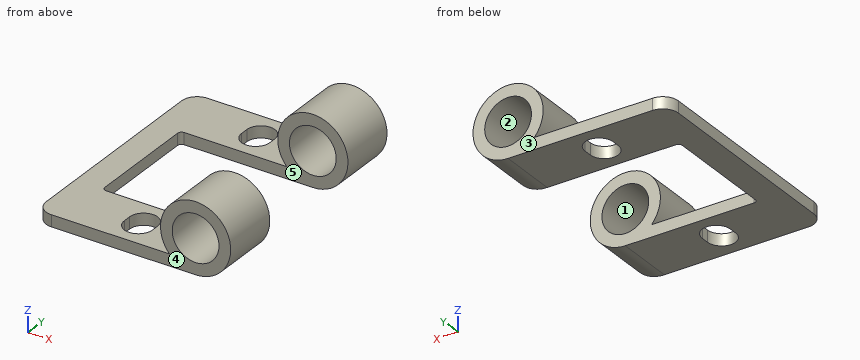
from build123d import *

# Parameters (mm, degrees)
SKETCH_2_W             = 16
SKETCH_2_H             = 30
SM_BASE_FLANGE_1_DEPTH = 1.5
SKETCH_7_R             = 4.5
SKETCH_7_R_2           = 3
EXTRUDE_1_DEPTH        = 30
SKETCH_8_W             = 1.5
SKETCH_8_H             = 7.5
EXTRUDE_1_2_DEPTH      = 4.5
SKETCH_9_W             = 25
SKETCH_9_H             = 15
CUT_EXTRUDE_1_DEPTH    = 41.074929819
FILLET_1_R             = 2
CUT_EXTRUDE_2_DEPTH    = 10
FILLET_2_R             = 0.5


# Sheet-metal steps are written as plain solids
with BuildPart() as part:
    # Sketch 2 → Базовая кромка1 (new body)
    with BuildSketch(Plane.XY):
        with Locations((8, -15)):
            Rectangle(SKETCH_2_W, SKETCH_2_H)
    extrude(amount=-SM_BASE_FLANGE_1_DEPTH)



with BuildPart() as body_2:
    # Эскиз7 → Extrude 1 (new body)
    with BuildSketch(Plane.XZ.offset(30)):
        with Locations((20.5, 3)):
            Circle(SKETCH_7_R)
        with Locations((20.5, 3)):
            Circle(SKETCH_7_R_2, mode=Mode.SUBTRACT)
    extrude(amount=-EXTRUDE_1_DEPTH)


with BuildPart() as part_1:
    add(part.part)

    add(body_2.part)  # Extrude 1 2 merges body 2
    # Эскиз8 → Extrude 1 2 (add)
    with BuildSketch(Plane(origin=(16, 0, 0), x_dir=(0, 0, -1), z_dir=(1, 0, 0))):
        with Locations((0.75, -26.25)):
            Rectangle(SKETCH_8_W, SKETCH_8_H)
        with Locations((0.75, -3.75)):
            Rectangle(SKETCH_8_W, SKETCH_8_H)
    extrude(amount=EXTRUDE_1_2_DEPTH)

    # Эскиз9 → Вырез-Вытянуть1 (cut, through all)
    with BuildSketch(Plane.XY.offset(-1.5)):
        with Locations((16, -15)):
            Rectangle(SKETCH_9_W, SKETCH_9_H)
    extrude(amount=CUT_EXTRUDE_1_DEPTH, mode=Mode.SUBTRACT)

    # Скругление1
    fillet_1_edges = [part_1.edges().sort_by_distance(p)[0] for p in [
        (0, 0, -0.75),
        (0, -30, -0.75),
    ]]
    fillet(fillet_1_edges, radius=FILLET_1_R)

    # Эскиз10 → Вырез-Вытянуть2 (cut)
    with BuildSketch(Plane.XY):
        with BuildLine():
            Line((9.2, -26.75), (9.2, -25.75))
            ThreePointArc((9.2, -25.75), (11, -23.95), (12.8, -25.75))
            Line((12.8, -25.75), (12.8, -26.75))
            ThreePointArc((12.8, -26.75), (11, -28.55), (9.2, -26.75))
        make_face()
        with BuildLine():
            Line((9.2, -3.25), (9.2, -4.25))
            ThreePointArc((9.2, -4.25), (11, -6.05), (12.8, -4.25))
            Line((12.8, -4.25), (12.8, -3.25))
            ThreePointArc((12.8, -3.25), (11, -1.45), (9.2, -3.25))
        make_face()
    extrude(amount=-CUT_EXTRUDE_2_DEPTH, mode=Mode.SUBTRACT)

    # Скругление2
    fillet_2_edges = [part_1.edges().sort_by_distance(p)[0] for p in [
        (3.5, -22.5, -0.75),
        (3.5, -7.5, -0.75),
    ]]
    fillet(fillet_2_edges, radius=FILLET_2_R)


solid = part_1.part
Model file for the job. Use its own axes, mm. Face numbers are marked on the shaded views. A direction names the side the tool comes from. Round coordinates to 2 decimals unless told otherwise and drop trailing zeros. Order: outer loops, then holes, each group sorted by start corner. A loop starts at its lowest first (then second) coordinate and runs counter-clockwise, first axis right, second up.
(1) Band-saw the part on C-C (z = 3). List the corners of the cut face in (x, y).
(2) Band-saw the part on D-D (x = 6). List the corners of the cut face in (y, z).
(3) 3-axis set-ups, long thin cutter, end or side, ignore diameter. For the marked faces 4 and 5: which of +Z, -Z, +X, -X, +Y, -Y reach the whole face in a straight line?
(4) Pull direction X, two halves, no side cores. Call the marked faces 1, 2 and 3: released by +X, released by -X, zero draft, split by the parting line, or undercut.
(5) Drill centre lines: line 1 (Z direction, x = 20.5, y = -27.5); line 2 (Y direction, x = 5.75, z = -1); line 3 (X direction, y = -26, z = 3). Where is each one in solid material? Low to high.
(6) Pin check, flat tips, straight feed: pin 1 (3 mm diameter, centred on x = 16, y = -24.5, fed in from +Z); pin 2 (0.8 mm diameter, centred on y = -18, z = -0.5, fed in from +X); pin 3 (0.5 mm diameter, centred on y = -4, z = -0.5, fed in from +X). Stop position of each tip, or through.
(7) Band-saw the part on A-A (y = -2.5). List the corners of the cut face in (x, z).
(8) Band-saw the part on B-B (x = 11). List the corners of the cut face in (y, z), then the cut area to 3 significant figures.
Verdict:
1. outline: (16, -30) - (17.5, -30) - (17.5, -22.5) - (16, -22.5) - close; (16, -7.5) - (17.5, -7.5) - (17.5, 0) - (16, 0) - close; (23.5, -30) - (25, -30) - (25, -22.5) - (23.5, -22.5) - close; (23.5, -7.5) - (25, -7.5) - (25, 0) - (23.5, 0) - close
2. outline: (-30, -1.5) - (-22.5, -1.5) - (-22.5, 0) - (-30, 0) - close; (-7.5, -1.5) - (0, -1.5) - (0, 0) - (-7.5, 0) - close
3. face 4: +Z, -Z, +X, -X, -Y
3. face 5: +Z, -Z, +X
4. face 1: undercut
4. face 2: undercut
4. face 3: zero draft
5. line 1: z = -1.5 to 0, 6 to 7.5
5. line 2: y = -30 to -22.5, -7.5 to 0
5. line 3: x = 16 to 17.5, 23.5 to 25
6. pin 1: stops at z = 6.35
6. pin 2: stops at x = 3.5
6. pin 3: stops at x = 23.61
7. outline: (0, -1.5) - (9.36, -1.5) - (9.36, 0) - (0, 0) - close; (12.64, -1.5) - (20.5, -1.5) arc R4.5 ccw (long way) to (17.15, 0) - (12.64, 0) - close; hole circle Ø6 at (20.5, 3)
8. outline: (-30, -1.5) - (-28.55, -1.5) - (-28.55, 0) - (-30, 0) - close; (-23.95, -1.5) - (-22.5, -1.5) - (-22.5, 0) - (-23.95, 0) - close; (-7.5, -1.5) - (-6.05, -1.5) - (-6.05, 0) - (-7.5, 0) - close; (-1.45, -1.5) - (0, -1.5) - (0, 0) - (-1.45, 0) - close
8. area: 8.70 mm2
